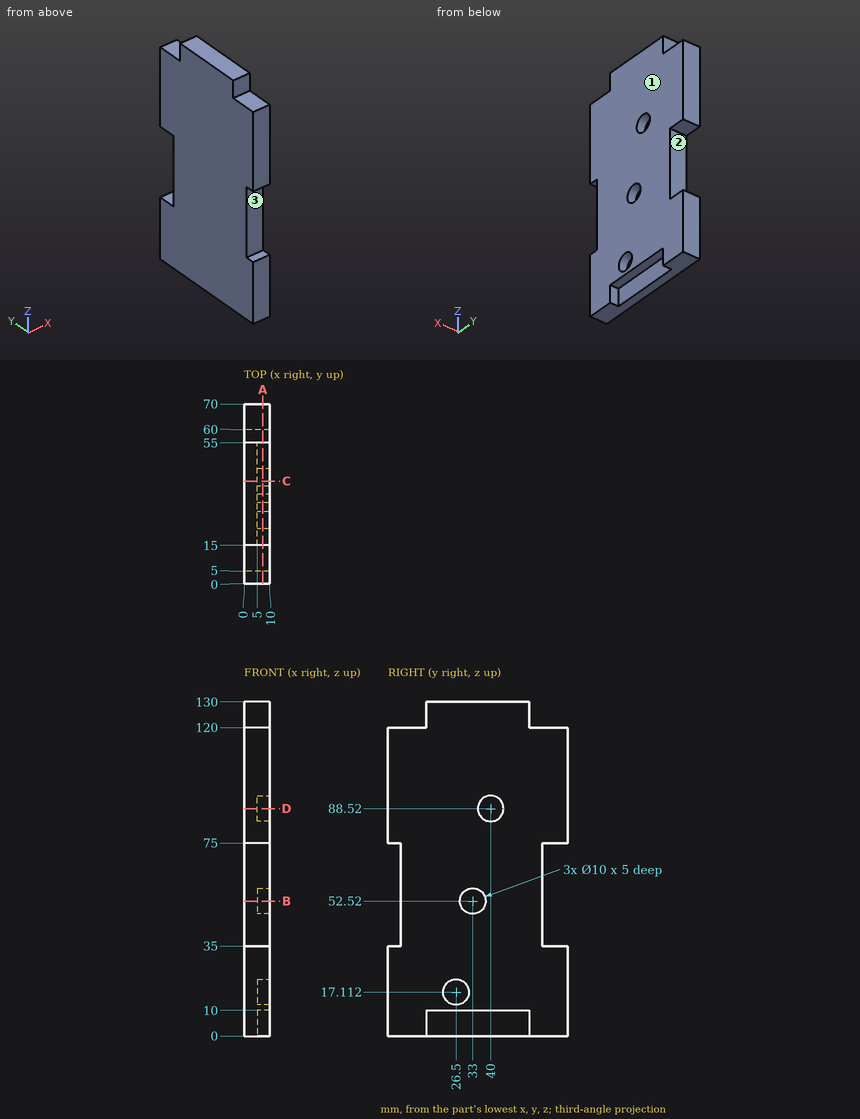
Geometry: see drawing. Coordinates: mm, zero at the bounding-box minimum. Coordinates: 2 decimals unless noted, no trailing zeros. Loops run counter-clockwise (first coordinate to the right, second up) from the corner with the lowest first, then second, coordinate; pieces in that order, holes last. Notation, with made-up numbers: (57, -31) -> (104, -31) arc R30 cw to (104, 4) -> close; hole circle Ø1 at (87.25, 76). An arc over 180 degrees is marked (long way). Use a Markdown table: item, result.
1) Cut plane C-C (y = 40). Return the cut outline in (x, z).
Results found:
| item | result |
|---|---|
| outline | (0, 0) -> (5, 0) -> (5, 10) -> (10, 10) -> (10, 83.52) -> (5, 83.52) -> (5, 93.52) -> (10, 93.52) -> (10, 130) -> (0, 130) -> close |
2) Pull-direction query (Z, two-part tool) for the marked faces 1, 2 and 3; classes: released by +Z, released by -Z, zero draft, split by the parting line, or undercut.
Results found:
| item | result |
|---|---|
| face 1 | zero draft |
| face 2 | undercut |
| face 3 | undercut |
3) Cut plane B-B (z = 52.52). Return the cut outline in (x, y).
Results found:
| item | result |
|---|---|
| outline | (0, 5) -> (10, 5) -> (10, 28) -> (5, 28) -> (5, 38) -> (10, 38) -> (10, 60) -> (0, 60) -> close |
4) Contact query for flat-ended pins moving along their axis: pin 1 (16 mm diameter, centred on y = 40, z = 88.52, fed in from -X); pin 2 (1.5 mm diameter, centred on x = 8, z = 41.5, fed in from -Y); pin 3 (5 mm diameter, centred on x = 3.5, z = 123, fed in from -Y); pin 4 (5.5 mm diameter, centred on x = 7, y = 1.5, fed in from +Z). Output: stop coordinate, or through.
Results found:
| item | result |
|---|---|
| pin 1 | stops at x = 0 |
| pin 2 | stops at y = 5 |
| pin 3 | stops at y = 15 |
| pin 4 | stops at z = 120 |
5) Material intervals for line 1 along Y through (x, z) = (6.45, 52.52); line 2 along Y through (x, z) = (7.5, 6); line 3 along Z through (x, y) = (9, 32.5) (1 decimal), sorted ascending. Write a range as from..to.
Results found:
| item | result |
|---|---|
| line 1 | y = 5..28, 38..60 |
| line 2 | y = 0..15, 55..70 |
| line 3 | z = 10..47.5, 57.5..130 |
6) Cut plane A-A (x = 7.25). Return the cut outline in (y, z), then the cut area to 3 significant figures.
Results found:
| item | result |
|---|---|
| outline | (0, 0) -> (15, 0) -> (15, 10) -> (55, 10) -> (55, 0) -> (70, 0) -> (70, 35) -> (60, 35) -> (60, 75) -> (70, 75) -> (70, 120) -> (55, 120) -> (55, 130) -> (15, 130) -> (15, 120) -> (0, 120) -> (0, 75) -> (5, 75) -> (5, 35) -> (0, 35) -> close; hole circle Ø10 at (26.5, 17.11); hole circle Ø10 at (33, 52.52); hole circle Ø10 at (40, 88.52) |
| area | 7,560 mm2 |
7) Cut plane D-D (z = 88.52). Return the cut outline in (x, y), then the cut area to 3 significant figures.
Results found:
| item | result |
|---|---|
| outline | (0, 0) -> (10, 0) -> (10, 35) -> (5, 35) -> (5, 45) -> (10, 45) -> (10, 70) -> (0, 70) -> close |
| area | 650 mm2 |
